from build123d import *

# Parameters (mm, degrees)
SKETCH1_W               = 190
SKETCH1_H               = 90
BOSS_EXTRUDE1_DEPTH     = 4
SKETCH2_R               = 1.75
CUT_EXTRUDE8_DEPTH      = 2
SKETCH14_R              = 1.75
CUT_EXTRUDE9_DEPTH      = 4
MIRROR9_COPY_1_SKETCH_R = 1.75
MIRROR9_COPY_1_DEPTH    = 2
MIRROR9_COPY_2_SKETCH_R = 1.75
MIRROR9_COPY_2_DEPTH    = 4
SKETCH16_W              = 70.6
SKETCH16_H              = 56
CUT_EXTRUDE10_DEPTH     = 2
CUT_EXTRUDE11_DEPTH     = 4
SKETCH18_W              = 50
SKETCH18_H              = 35
CUT_EXTRUDE12_DEPTH     = 4
SKETCH19_W              = 9
SKETCH19_H              = 21.5
BOSS_EXTRUDE2_DEPTH     = 2
CUT_EXTRUDE13_DEPTH     = 6
FILLET1_R               = 10
SKETCH21_W              = 4.7
SKETCH21_H              = 13
CUT_EXTRUDE14_DEPTH     = 2
SKETCH22_W              = 20
SKETCH22_H              = 15
CUT_EXTRUDE15_DEPTH     = 4
SKETCH23_W              = 4.7
SKETCH23_H              = 11
CUT_EXTRUDE16_DEPTH     = 2


with BuildPart() as part:
    # Sketch1 → Boss-Extrude1 (new body)
    with BuildSketch(Plane(origin=(0, 0, 0), x_dir=(1, 0, 0), z_dir=(0, 1, 0))):
        Rectangle(SKETCH1_W, SKETCH1_H)
    extrude(amount=BOSS_EXTRUDE1_DEPTH)

    # Sketch2 → Cut-Extrude8 (cut)
    with BuildSketch(Plane(origin=(0, 4, 0), x_dir=(1, 0, 0), z_dir=(0, 1, 0))):
        Polygon((-84.935953931, 38), (-86.525120789, 40.752517739), (-89.703454503, 40.752517739), (-91.292621361, 38), (-89.703454503, 35.247482261), (-86.525120789, 35.247482261), align=None)
        with Locations(Location((-88.114287646, 38, 0), (0, 0, 270))):
            Circle(SKETCH2_R, mode=Mode.SUBTRACT)
    cut_extrude8 = extrude(amount=-CUT_EXTRUDE8_DEPTH, mode=Mode.SUBTRACT)

    # Sketch14 → Cut-Extrude9 (cut)
    with BuildSketch(Plane(origin=(0, 4, 0), x_dir=(1, 0, 0), z_dir=(0, 1, 0))):
        with Locations(Location((-88.114287646, 38, 0), (0, 0, 270))):
            Circle(SKETCH14_R)
    cut_extrude9 = extrude(amount=-CUT_EXTRUDE9_DEPTH, mode=Mode.SUBTRACT)

    # Mirror8: Cut-Extrude8, Cut-Extrude9 across plane
    add(cut_extrude8.mirror(Plane.XY), mode=Mode.SUBTRACT)
    add(cut_extrude9.mirror(Plane.XY), mode=Mode.SUBTRACT)

    # Mirror9: Cut-Extrude8, Cut-Extrude9 across plane
    add(cut_extrude8.mirror(Plane(origin=(0, 0, 0), x_dir=(0, 0, 1), z_dir=(1, 0, 0))), mode=Mode.SUBTRACT)
    add(cut_extrude9.mirror(Plane(origin=(0, 0, 0), x_dir=(0, 0, 1), z_dir=(1, 0, 0))), mode=Mode.SUBTRACT)

    # Mirror9 copy 1 sketch → Mirror9 copy 1 (cut)
    with BuildSketch(Plane(origin=(0, 4, 0), x_dir=(-1, 0, 0), z_dir=(0, 1, 0))):
        Polygon((-84.935953931, 38), (-86.525120789, 40.752517739), (-89.703454503, 40.752517739), (-91.292621361, 38), (-89.703454503, 35.247482261), (-86.525120789, 35.247482261), align=None)
        with Locations(Location((-88.114287646, 38, 0), (0, 0, 270))):
            Circle(MIRROR9_COPY_1_SKETCH_R, mode=Mode.SUBTRACT)
    extrude(amount=-MIRROR9_COPY_1_DEPTH, mode=Mode.SUBTRACT)

    # Mirror9 copy 2 sketch → Mirror9 copy 2 (cut)
    with BuildSketch(Plane(origin=(0, 4, 0), x_dir=(-1, 0, 0), z_dir=(0, 1, 0))):
        with Locations(Location((-88.114287646, 38, 0), (0, 0, 270))):
            Circle(MIRROR9_COPY_2_SKETCH_R)
    extrude(amount=-MIRROR9_COPY_2_DEPTH, mode=Mode.SUBTRACT)

    # Sketch16 → Cut-Extrude10 (cut)
    with BuildSketch(Plane.XZ):
        with Locations((-55, 0)):
            Rectangle(SKETCH16_W, SKETCH16_H)
    extrude(amount=-CUT_EXTRUDE10_DEPTH, mode=Mode.SUBTRACT)

    # Sketch17 → Cut-Extrude11 (cut)
    with BuildSketch(Plane.XZ.offset(-2)):
        with BuildLine():
            Line((-77.910700379, -21.65), (-67.489299621, -21.65))
            ThreePointArc((-67.489299621, -21.65), (-65.139299621, -24), (-67.489299621, -26.35))
            Line((-67.489299621, -26.35), (-77.910700379, -26.35))
            ThreePointArc((-77.910700379, -26.35), (-80.260700379, -24), (-77.910700379, -21.65))
        make_face()
        with BuildLine():
            Line((-24.7, -17.749516727), (-24.7, -7.749516727))
            ThreePointArc((-24.7, -7.749516727), (-22.7, -5.749516727), (-20.7, -7.749516727))
            Line((-20.7, -7.749516727), (-20.7, -17.749516727))
            ThreePointArc((-20.7, -17.749516727), (-22.7, -19.749516727), (-24.7, -17.749516727))
        make_face()
        with BuildLine():
            Line((-20.7, 22.876592803), (-20.7, 9.624373743))
            ThreePointArc((-20.7, 9.624373743), (-22.7, 7.624373743), (-24.7, 9.624373743))
            Line((-24.7, 9.624373743), (-24.7, 22.876592803))
            ThreePointArc((-24.7, 22.876592803), (-22.7, 24.876592803), (-20.7, 22.876592803))
        make_face()
    extrude(amount=-CUT_EXTRUDE11_DEPTH, mode=Mode.SUBTRACT)

    # Sketch18 → Cut-Extrude12 (cut)
    with BuildSketch(Plane.XZ.offset(-2)):
        with Locations((-55, 0)):
            Rectangle(SKETCH18_W, SKETCH18_H)
    extrude(amount=-CUT_EXTRUDE12_DEPTH, mode=Mode.SUBTRACT)

    # Sketch19 → Boss-Extrude2 (add)
    with BuildSketch(Plane.XZ):
        with Locations((-12.75, -25)):
            Rectangle(SKETCH19_W, SKETCH19_H)
        with Locations((22.75, -25)):
            Rectangle(SKETCH19_W, SKETCH19_H)
    extrude(amount=BOSS_EXTRUDE2_DEPTH)

    # Sketch20 → Cut-Extrude13 (cut)
    with BuildSketch(Plane.XZ.offset(2)):
        with BuildLine():
            Line((-14.75, -32.5), (-14.75, -17.5))
            ThreePointArc((-14.75, -17.5), (-12.75, -15.5), (-10.75, -17.5))
            Line((-10.75, -17.5), (-10.75, -32.5))
            ThreePointArc((-10.75, -32.5), (-12.75, -34.5), (-14.75, -32.5))
        make_face()
        with BuildLine():
            Line((24.75, -32.5), (24.75, -17.5))
            ThreePointArc((24.75, -17.5), (22.75, -15.5), (20.75, -17.5))
            Line((20.75, -17.5), (20.75, -32.5))
            ThreePointArc((20.75, -32.5), (22.75, -34.5), (24.75, -32.5))
        make_face()
    extrude(amount=-CUT_EXTRUDE13_DEPTH, mode=Mode.SUBTRACT)

    # Fillet1
    fillet1_edges = [part.edges().sort_by_distance(p)[0] for p in [
        (-95, 2, 45),
        (-95, 2, -45),
        (95, 2, -45),
        (95, 2, 45),
    ]]
    fillet(fillet1_edges, radius=FILLET1_R)

    # Sketch21 → Cut-Extrude14 (cut)
    with BuildSketch(Plane.XZ):
        with Locations((-92.65, 12.5)):
            Rectangle(SKETCH21_W, SKETCH21_H)
    extrude(amount=-CUT_EXTRUDE14_DEPTH, mode=Mode.SUBTRACT)

    # Sketch22 → Cut-Extrude15 (cut)
    with BuildSketch(Plane.XZ):
        with Locations((5, -25)):
            Rectangle(SKETCH22_W, SKETCH22_H)
    extrude(amount=-CUT_EXTRUDE15_DEPTH, mode=Mode.SUBTRACT)

    # Sketch23 → Cut-Extrude16 (cut)
    with BuildSketch(Plane.XZ):
        with Locations((-92.65, -17.5)):
            Rectangle(SKETCH23_W, SKETCH23_H)
    extrude(amount=-CUT_EXTRUDE16_DEPTH, mode=Mode.SUBTRACT)


solid = part.part
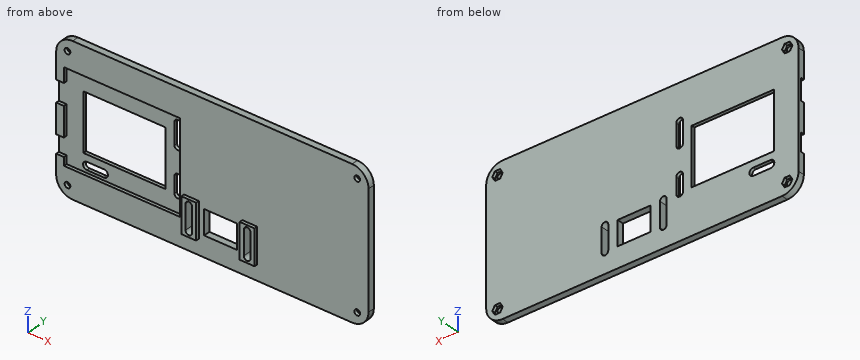
The model under review builds one solid part; all positions refer to its coordinate system, in mm. Round coordinates to 2 decimals unless told otherwise and drop trailing zeros. Write each loop counter-clockwise with the first axis right and the second up, starting at its lowest first coordinate (ties: lowest second). Pieces come first, ordered by that corner, then holes. Notation, with made-up numbers: M -23.75,48.5 L 31.25,48.5 A25 ccw 31.25,67.5 Z; hole C 65,54 d6. An arc over 180 degrees is marked long. Answer as CSV lines item,"result". Start each with the question number.
Q1. Clearance check with flat-ended pins moving along their axes: P1, Ø1.6, axis at x = 24, y = -1, coming from the +Z side; P2, Ø2, axis at x = -88, y = 3.5, coming from the +Z side; P3, Ø5, axis at x = 53, z = 1, coming from the -Y side. State where each tip first meets the part, or that it passes through.
Q2. Wall thickness on line 1 along X through (y, z) = (2.1, -8.5); line 2 along X through (y, z) = (1.1, 38); line 3 along Z through (x, y) = (-13, 0.5): over which ranges is each line inside the solid? List them lowest first.
Q3. Consider section C-C, the plane x = 77. Give the boundary of the cut face in (y, z).
Q4. Consider section A-A, the plane x = -55. Give the boundary of the cut face in (y, z).
Q5. Consider section B-B, the plane x = -22.7. Give the boundary of the cut face in (y, z).
Result set:
1,P1,"stops at z = -14.25"
1,P2,"stops at z = 44.8"
1,P3,"stops at y = 0"
2,line 1,"x = -95 to -80, -30 to -24.7, -20.7 to 95"
2,line 2,"x = -94.54 to -89.86, -86.36 to 86.36, 89.86 to 94.54"
2,line 3,"z = -45 to -34.48, -15.52 to 45"
3,outline,"M 0,-45 L 4,-45 L 4,45 L 0,45 Z"
4,outline,"M 0,-45 L 4,-45 L 4,-17.5 L 2,-17.5 L 2,-28 L 0,-28 Z; M 0,28 L 2,28 L 2,17.5 L 4,17.5 L 4,45 L 0,45 Z"
5,outline,"M 0,-45 L 4,-45 L 4,-19.75 L 2,-19.75 L 2,-28 L 0,-28 Z; M 0,28 L 2,28 L 2,24.88 L 4,24.88 L 4,45 L 0,45 Z; M 2,-5.75 L 4,-5.75 L 4,7.62 L 2,7.62 Z"
